Autodesk Inventor part; units mm, degrees
ref_plane "YZ Plane" through (0, 0, 0) normal (1, 0, 0) x (0, 1, 0)
ref_plane "XZ Plane" through (0, 0, 0) normal (0, 1, 0) x (-1, 0, 0)
ref_plane "XY Plane" through (0, 0, 0) normal (0, 0, 1) x (1, 0, 0)
sketch "Sketch2" plane through (0, 0, 0) normal (0, 0, 1) x (1, 0, 0)
  arc A0 (93, -22.6) -> (97, -22.6) centre (95, -22.6) ccw construction
  arc A1 (97, -22.6) -> (93, -22.6) centre (95, -22.6) ccw construction
  arc A2 (97, 22.6) -> (93, 22.6) centre (95, 22.6) ccw construction
  arc A3 (93, 22.6) -> (97, 22.6) centre (95, 22.6) ccw construction
  line L0 (207.9, 0) -> (-207.9, 0) construction
  line L1 (0, -294.0706) -> (0, 294.0706) construction
  line L2 (87, -30.6) -> (103, -30.6)
  line L3 (105, -28.6) -> (105, 34)
  line L4 (103, 36) -> (71, 36)
  line L5 (69, 34) -> (69, -12)
  line L6 (71, -14) -> (83, -14)
  line L7 (85, -16) -> (85, -28.6)
  arc A4 (103, -30.6) -> (105, -28.6) centre (103, -28.6) ccw
  arc A5 (85, -28.6) -> (87, -30.6) centre (87, -28.6) ccw
  arc A6 (85, -16) -> (83, -14) centre (83, -16) ccw
  arc A7 (69, -12) -> (71, -14) centre (71, -12) ccw
  arc A8 (71, 36) -> (69, 34) centre (71, 34) ccw
  arc A9 (105, 34) -> (103, 36) centre (103, 34) ccw
  circle A10 centre (78, -7.2) radius 2.05
  circle A11 centre (78, 14.8) radius 2.05
  circle A12 centre (78, 28.8) radius 2.05
  line L8 (78, -7.2) -> (78, 28.8) construction
  line L9 (98, -18.65) -> (98, -26.55) construction
  line L10 (98, -26.55) -> (92, -26.55) construction
  line L11 (92, -18.65) -> (92, -26.55) construction
  line L12 (98, -18.65) -> (92, -18.65) construction
  arc A13 (97, -22.6) -> (93, -22.6) centre (95, -22.6) ccw construction
  arc A14 (93, -22.6) -> (97, -22.6) centre (95, -22.6) ccw construction
  line L13 (92, 18.65) -> (92, 26.55) construction
  line L14 (92, 26.55) -> (98, 26.55) construction
  line L15 (98, 18.65) -> (98, 26.55) construction
  line L16 (92, 18.65) -> (98, 18.65) construction
  arc A15 (93, 22.6) -> (97, 22.6) centre (95, 22.6) ccw construction
  arc A16 (97, 22.6) -> (93, 22.6) centre (95, 22.6) ccw construction
  arc A17 (97, -22.6) -> (93, -22.6) centre (95, -22.6) ccw construction
  arc A18 (97.4356, -1.2768) -> (97.4356, 1.2768) centre (95, 0) ccw construction
  circle A19 centre (95, 0) radius 2.05
  circle A20 centre (95, 22.6) radius 2.05
  circle A21 centre (95, -22.6) radius 2.05
  point P0 (0, 0)
  point P1 (105, 36)
  point P2 (69, 36)
extrude "Extrusion2" add sketch "Sketch2" along normal blind 1.5
properties part number "Oxy_cut" material "Stainless Steel"
Work out the finished part from the listing and answer in its coordinate system (mm). A direction names the side the tool comes from. Coordinates: 2 decimals unless noted, no trailing zeros. Loops run counter-clockwise (first coordinate to the right, second up) from the corner with the lowest first, then second, coordinate; pieces in that order, holes last. Notation, with made-up numbers: (78, 49) -> (89, 49) arc R16 ccw to (89, 63) -> close; hole circle Ø11 at (-9.5, 66). An arc over 180 degrees is marked (long way). Answer as CSV lines item,"result".
Q1. The part is cut by section C-C on z = 0.35. Write down the section's boundary in (x, y), and give its area (3 significant figures).
Findings:
outline,"(69, -12) arc R2 ccw to (71, -14) -> (83, -14) arc R2 cw to (85, -16) -> (85, -28.6) arc R2 ccw to (87, -30.6) -> (103, -30.6) arc R2 ccw to (105, -28.6) -> (105, 34) arc R2 ccw to (103, 36) -> (71, 36) arc R2 ccw to (69, 34) -> close; hole circle Ø4.1 at (78, -7.2); hole circle Ø4.1 at (78, 14.8); hole circle Ø4.1 at (78, 28.8); hole circle Ø4.1 at (95, -22.6); hole circle Ø4.1 at (95, 0); hole circle Ø4.1 at (95, 22.6)"
area,"2,050 mm²"
Q2. The part is cut by section A-A on x = 95. Write down the section's boundary in (y, z), and give its area (4 significant figures).
Findings:
outline,"(-30.6, 0) -> (-24.65, 0) -> (-24.65, 1.5) -> (-30.6, 1.5) -> close; (-20.55, 0) -> (-2.05, 0) -> (-2.05, 1.5) -> (-20.55, 1.5) -> close; (2.05, 0) -> (20.55, 0) -> (20.55, 1.5) -> (2.05, 1.5) -> close; (24.65, 0) -> (36, 0) -> (36, 1.5) -> (24.65, 1.5) -> close"
area,"81.45 mm²"
Q3. Find the intervals of material crossed by probe 1 along Y at (x, z) = (78, 0.4); probe 2 along Y at (x, z) = (95, 1); probe 3 along X at (y, z) = (23, 1.05), in increasing order.
Findings:
probe 1,"y = -14 to -9.25, -5.15 to 12.75, 16.85 to 26.75, 30.85 to 36"
probe 2,"y = -30.6 to -24.65, -20.55 to -2.05, 2.05 to 20.55, 24.65 to 36"
probe 3,"x = 69 to 92.99, 97.01 to 105"
Q4. Each of these flat-tipped pins is pushed along its axis until it touches: pin 1 (3.5 mm diameter, centred on x = 78, y = 28.8, fed in from -Z); pin 2 (0.8 mm diameter, centred on y = -21, z = 0.5, fed in from -X); pin 3 (0.8 mm diameter, centred on x = 78.5, z = 0.5, fed in from -Y). Where does it stop, or does it pass through?
Findings:
pin 1,"passes through"
pin 2,"stops at x = 85"
pin 3,"stops at y = -14"
Q5. The part is cut by section D-D on x = 78. Write down the section's boundary in (y, z).
Findings:
outline,"(-14, 0) -> (-9.25, 0) -> (-9.25, 1.5) -> (-14, 1.5) -> close; (-5.15, 0) -> (12.75, 0) -> (12.75, 1.5) -> (-5.15, 1.5) -> close; (16.85, 0) -> (26.75, 0) -> (26.75, 1.5) -> (16.85, 1.5) -> close; (30.85, 0) -> (36, 0) -> (36, 1.5) -> (30.85, 1.5) -> close"
Q6. A tool of negligible diameter and unlimited length cuts with its end or side. For faces 4 (the face through (85, -22, 1)), 5 (the face through (69, 11, 1)), from which of +Z, -Z, +X, -X, +Y, -Y can it reach the whole face along a straight path? Write none if from no direction.
Findings:
face 4,"+Z, -Z, -X, -Y"
face 5,"+Z, -Z, -X, +Y, -Y"
Q7. The part is cut by section B-B on y = -22.6. Write down the section's boundary in (x, z).
Findings:
outline,"(85, 0) -> (92.95, 0) -> (92.95, 1.5) -> (85, 1.5) -> close; (97.05, 0) -> (105, 0) -> (105, 1.5) -> (97.05, 1.5) -> close"
Q8. For a pull along X with two mould halves and no side action, classify faces 1 (the face through (75.95, 14.71, 0.74)), 2 (the face through (77, -14, 1)), 3 (the face through (104.4, 35.43, 0.74)) as +X half, -X half, draft (parallel to the pull), parting line (faces both ways), or undercut.
Findings:
face 1,"undercut"
face 2,"draft"
face 3,"+X half"
